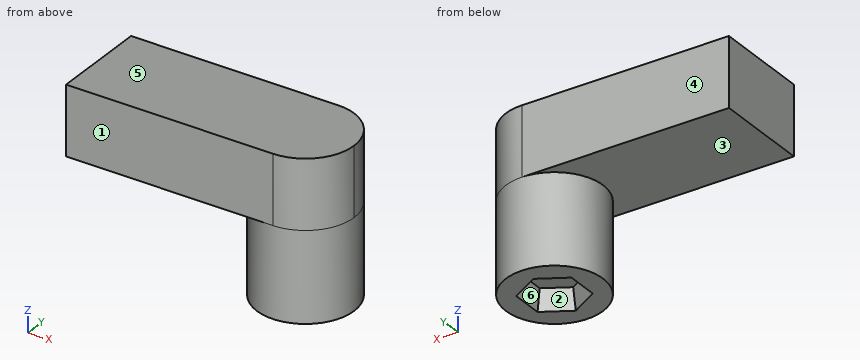
from build123d import *

# Parameters (mm, degrees)
F0_R     = 7.0414518843
F1_DEPTH = 3
F2_R     = 7.0414518843
F3_DEPTH = 10
F5_DEPTH = 10
F6_SIZE2 = 2.99999
F6_SIZE  = 0.49999


# Not quite as in the source:
# - a fillet or chamfer is up to 0.001 mm smaller than in the source, because OpenCascade refuses the exact size


with BuildPart() as f1:
    # F0 (on Top) → F1 (new body)
    with BuildSketch(Plane.XY):
        Circle(F0_R)
        Polygon((0, -4.0414518843), (-3.5, -2.0207259422), (-3.5, 2.0207259422), (0, 4.0414518843), (3.5, 2.0207259422), (3.5, -2.0207259422), align=None, mode=Mode.SUBTRACT)
    extrude(amount=F1_DEPTH)

    # F2 (on face) → F3 (join)
    with BuildSketch(Plane.XY.offset(3)):
        Circle(F2_R)
        Polygon((3.5, -2.0207259422), (0, -4.0414518843), (-3.5, -2.0207259422), (-3.5, 2.0207259422), (0, 4.0414518843), (3.5, 2.0207259422), align=None, mode=Mode.SUBTRACT)
        Polygon((-3.5, -2.0207259422), (0, -4.0414518843), (3.5, -2.0207259422), (3.5, 2.0207259422), (0, 4.0414518843), (-3.5, 2.0207259422), align=None)
    extrude(amount=F3_DEPTH)

    # F4 (on face) → F5 (join)
    with BuildSketch(Plane.XY.offset(13)):
        with BuildLine():
            ThreePointArc((7.0414518843, 0), (4.9790583768, 4.9790583768), (0, 7.0414518843))
            ThreePointArc((0, 7.0414518843), (-7.0414518843, 0), (0, -7.0414518843))
            ThreePointArc((0, -7.0414518843), (4.9790583768, -4.9790583768), (7.0414518843, 0))
        make_face()
        with BuildLine():
            ThreePointArc((0, -7.0414518843), (-7.0414518843, 0), (0, 7.0414518843))
            Line((0, 7.0414518843), (-30, 7.0414518843))
            Line((-30, 7.0414518843), (-30, -7.0414518843))
            Line((-30, -7.0414518843), (0, -7.0414518843))
        make_face()
    extrude(amount=F5_DEPTH)

    # F6 (size 0.5 and 3 in the source; OpenCascade refuses exactly that, so slightly less here)
    f6_edges = [f1.edges().sort_by_distance(p)[0] for p in [
        (-1.75, -3.031089, 0),
        (-3.5, 0, 0),
        (1.75, -3.031089, 0),
        (3.5, 0, 0),
        (1.75, 3.031089, 0),
        (-1.75, 3.031089, 0),
    ]]
    f6_side = f1.faces().sort_by_distance((-6.84229, 0, 0))[0]
    chamfer(f6_edges, length=F6_SIZE, length2=F6_SIZE2, reference=f6_side)


solid = f1.part
The listing builds one solid part. Answer for the finished solid, in the listing's coordinates (mm). Face numbers are marked on the shaded views. A direction names the side the tool comes from. Round coordinates to 2 decimals unless told otherwise and drop trailing zeros. Write each loop counter-clockwise with the first axis right and the second up, starting at its lowest first coordinate (ties: lowest second). Pieces come first, ordered by that corner, then holes. Notation, with made-up numbers: M 68,-20.5 L 84,-20.5 A18 ccw 84,11.5 Z; hole C 60,-37.5 d1. An arc over 180 degrees is marked long. Write each question's results on one line, items separated by ' | '. Start each with the question number.
Item 1: A cutting plane is placed at C-C on x = -9.5. Write down the section's boundary in (y, z), and give its area (3 significant figures).
Item 2: Straight lines are drawn through the part: L1, parallel to Z at x = -19, y = -1; L2, parallel to Z at x = 0, y = -0.5; L3, parallel to X at y = -0.25, z = 11. For each, find the intervals that lie inside material, in ascending order. Write a range as [from, to].
Item 3: For a pull along Y with two mould halves and no side action, classify the marked faces 1, 2, 3 and 4 as pulls with the +Y half, pulls with the -Y half, needs draft (parallel to the pull), parting line crosses it, or undercut.
Item 4: A cutting plane is placed at A-A on y = 5.25. Write down the section's boundary in (x, z), and give its area (3 significant figures).
Item 5: Flat-ended cylindrical pins translate along their axes: pin 1 Ø1 at (y, z) = (-2, 5.5) entering from -X; pin 2 Ø8 at (y, z) = (-5, 5.5) entering from -X; pin 3 Ø2 at (y, z) = (3.5, 16.5) entering from +X. Find the tip coordinate at first contact, or state that the pin passes through.
Item 6: A cutting plane is placed at B-B on z = 17.5. Write down the section's boundary in (x, y).
Item 7: For the marked faces 5 and 6, determine the directions among +Z, -Z, +X, -X, +Y, -Y from which every point of the face is accessible in a straight line to the end or side of a thin tool.
Check sheet entries:
1) outline: M -7.04,13 L 7.04,13 L 7.04,23 L -7.04,23 Z | area: 141 mm²
2) L1: [13, 23] | L2: [3, 23] | L3: [-7.04, 7.04]
3) face 1: pulls with the -Y half | face 2: undercut | face 3: needs draft | face 4: pulls with the +Y half
4) outline: M -30,13 L -4.69,13 L -4.69,0 L 4.69,0 L 4.69,23 L -30,23 Z | area: 469 mm²
5) pin 1: x = -6.88 | pin 2: x = -6.97 | pin 3: x = 6.58
6) outline: M -30,-7.04 L 0,-7.04 A7.04 ccw 0,7.04 L -30,7.04 Z
7) face 5: +Z, +X, -X, +Y, -Y | face 6: -Z
